from build123d import *

# Parameters (mm, degrees)
F1_DEPTH = 60
F2_DEPTH = 25


# Not quite as in the source:
# - the program builds the solid bodies; features that only make, move or delete a surface that nothing else refers to are left out


with BuildPart() as f1:
    # F0 (on Top) → F1 (new body)
    with BuildSketch(Plane.XY):
        with BuildLine():
            ThreePointArc((-305.0224336339, -246.0090226419), (-425.7668614501, -572.66743243), (-365.4684518499, -915.6674839367))
            Line((-365.4684518499, -915.6674839367), (-337.7260933976, -915.6674839367))
            ThreePointArc((-337.7260933976, -915.6674839367), (-383.1853890072, -472.5820879471), (-129.4684518499, -106.4961260526))
            ThreePointArc((-129.4684518499, -106.4961260526), (-213.2726615111, 23.7464933662), (-249.4684518499, 174.3325160633))
            Line((-249.4684518499, 174.3325160633), (-249.4684518499, 474.3325160633))
            Line((-249.4684518499, 474.3325160633), (-278.4684518499, 474.3325160633))
            ThreePointArc((-278.4684518499, 474.3325160633), (-327.0089672753, 193.5023169021), (-280.3739250896, -87.6505867625))
            ThreePointArc((-280.3739250896, -87.6505867625), (-274.0048617812, -169.7394217084), (-305.0224336339, -246.0090226419))
        make_face()
        with BuildLine():
            ThreePointArc((-129.4684518499, -106.4961260526), (-383.1853890072, -472.5820879471), (-337.7260933976, -915.6674839367))
            Line((-337.7260933976, -915.6674839367), (-307.8033710716, -915.6674839367))
            ThreePointArc((-307.8033710716, -915.6674839367), (-322.9497717837, -884.2710326331), (-336.294380675, -852.0674300004))
            ThreePointArc((-336.294380675, -852.0674300004), (-349.0076832074, -449.9968879223), (-110.6437650385, -125.9521512216))
            ThreePointArc((-110.6437650385, -125.9521512216), (-120.198249318, -116.3616671102), (-129.4684518499, -106.4961260526))
        make_face()
        with BuildLine():
            ThreePointArc((-336.294380675, -852.0674300004), (-322.9497717837, -884.2710326331), (-307.8033710716, -915.6674839367))
            Line((-307.8033710716, -915.6674839367), (471.5315481501, -915.6674839367))
            Line((471.5315481501, -915.6674839367), (471.5315481501, -255.6674839367))
            Line((471.5315481501, -255.6674839367), (399.6472072601, -255.6674839367))
            Line((399.6472072601, -255.6674839367), (399.6472072601, -752.0674300004))
            ThreePointArc((399.6472072601, -752.0674300004), (370.3578853788, -822.778108119), (299.6472072601, -852.0674300004))
            Line((299.6472072601, -852.0674300004), (-336.294380675, -852.0674300004))
        make_face()
        with BuildLine():
            ThreePointArc((-249.4684518499, 174.3325160633), (-213.2726615111, 23.7464933662), (-129.4684518499, -106.4961260526))
            ThreePointArc((-129.4684518499, -106.4961260526), (-120.198249318, -116.3616671102), (-110.6437650385, -125.9521512216))
            ThreePointArc((-110.6437650385, -125.9521512216), (134.8677667197, -26.0001986196), (399.6472072601, -38.5760851606))
            Line((399.6472072601, -38.5760851606), (399.6472072601, -255.6674839367))
            Line((399.6472072601, -255.6674839367), (471.5315481501, -255.6674839367))
            Line((471.5315481501, -255.6674839367), (471.5315481501, 474.3325160633))
            Line((471.5315481501, 474.3325160633), (-249.4684518499, 474.3325160633))
            Line((-249.4684518499, 474.3325160633), (-249.4684518499, 174.3325160633))
        make_face()
    extrude(amount=F1_DEPTH)

    # F0 (on Top) → F2 (join)
    with BuildSketch(Plane.XY):
        with BuildLine():
            ThreePointArc((-110.6437650385, -125.9521512216), (-349.0076832074, -449.9968879223), (-336.294380675, -852.0674300004))
            Line((-336.294380675, -852.0674300004), (299.6472072601, -852.0674300004))
            ThreePointArc((299.6472072601, -852.0674300004), (370.3578853788, -822.778108119), (399.6472072601, -752.0674300004))
            Line((399.6472072601, -752.0674300004), (399.6472072601, -255.6674839367))
            Line((399.6472072601, -255.6674839367), (171.5315481501, -255.6674839367))
            ThreePointArc((171.5315481501, -255.6674839367), (19.2512340542, -215.1576843257), (-110.6437650385, -125.9521512216))
        make_face()
        with BuildLine():
            ThreePointArc((399.6472072601, -38.5760851606), (134.8677667197, -26.0001986196), (-110.6437650385, -125.9521512216))
            ThreePointArc((-110.6437650385, -125.9521512216), (19.2512340542, -215.1576843257), (171.5315481501, -255.6674839367))
            Line((171.5315481501, -255.6674839367), (399.6472072601, -255.6674839367))
            Line((399.6472072601, -255.6674839367), (399.6472072601, -38.5760851606))
        make_face()
    extrude(amount=F2_DEPTH)


solid = f1.part
Model file for the job. Use its own axes, mm. A direction names the side the tool comes from. Give positions to 0.01 mm unless a question says otherwise; leave off trailing zeros. Order: outer loops, then holes, each group sorted by start corner. A loop starts at its lowest first (then second) coordinate and runs counter-clockwise, first axis right, second up. Notation, with made-up numbers: (-16, -10) - (0, -10) arc R19 cw to (0, 11) - close; hole circle Ø5 at (-32, 6). An arc over 180 degrees is marked (long way). Return JSON: item names as keys, results as strings.
1) Cut at C-C, the plane x = 223. Give the cut face in (y, z), plus the area to 3 significant figures.
Geometry says:
{"outline": "(-915.67, 0) - (474.33, 0) - (474.33, 60) - (-17.37, 60) - (-17.37, 25) - (-852.07, 25) - (-852.07, 60) - (-915.67, 60) - close", "area": "54,200 mm²"}
2) Cut at D-D, the plane y = 4.5. Give the cut face in (x, z).
Geometry says:
{"outline": "(-306.47, 0) - (471.53, 0) - (471.53, 60) - (-306.47, 60) - close"}
3) Pull direction Y, two halves, no side cores. Call faces 1 (the cylindrical face through (-326.986, 197.511, 29.58)), 2 (the flat face through (102, 474.333, 30)), 3 (the flat face through (47, -915.667, 30)): pulls with the +Y half, pulls with the -Y half, needs draft (parallel to the pull), parting line crosses it, or undercut.
Geometry says:
{"face 1": "undercut", "face 2": "pulls with the +Y half", "face 3": "pulls with the -Y half"}
4) Cut at A-A, the plane z = 40. Give the cut face in (x, y), plus the area to 3 significant figures.
Geometry says:
{"outline": "(-365.47, -915.67) - (471.53, -915.67) - (471.53, 474.33) - (-278.47, 474.33) arc R853.38 ccw to (-280.37, -87.65) arc R179.17 cw to (-305.02, -246.01) arc R667.21 ccw to start; hole (-336.29, -852.07) - (299.65, -852.07) arc R100 ccw to (399.65, -752.07) - (399.65, -38.58) arc R615.48 ccw to start", "area": "580,000 mm²"}
5) Cut at B-B, the plane y = -318. Give the cut face in (x, z), plus the area to 3 significant figures.
Geometry says:
{"outline": "(-349.62, 0) - (471.53, 0) - (471.53, 60) - (399.65, 60) - (399.65, 25) - (-290.23, 25) - (-290.23, 60) - (-349.62, 60) - close", "area": "25,100 mm²"}
6) Flat gauge pins, fed straight in: P1, Ø3, axis at y = -313.5, z = 39, coming from the -X side; P2, Ø10.5, axis at y = -486.5, z = 48, coming from the -X side; P3, Ø2, axis at y = -145, z = 25.5, coming from the -X side. Where does each tip first touch, or does it go through?
Geometry says:
{"P1": "x = -348", "P2": "x = -413.42", "P3": "x = -271.91"}
7) Probe line 1 (Z direction, x = -36.5, y = -814.5); line 2 (Y direction, x = -256, z = 27); line 3 (X direction, y = -2, z = 50.5). List the from-to ranges inside material, lowest first. Write a range as from..to.
Geometry says:
{"line 1": "0..25", "line 2": "-915.67..-852.07, -266.53..474.33", "line 3": "-304.99..471.53"}
8) 3-axis set-ups, long thin cutter, end or side, ignore diameter. For faces 4 (the flat face through (6, -429, 25)), 5 (the flat face through (15, -211, 0)): which of +Z, -Z, +X, -X, +Y, -Y reach the whole face in a straight line?
Geometry says:
{"face 4": "+Z", "face 5": "-Z, +X, -X, +Y, -Y"}
